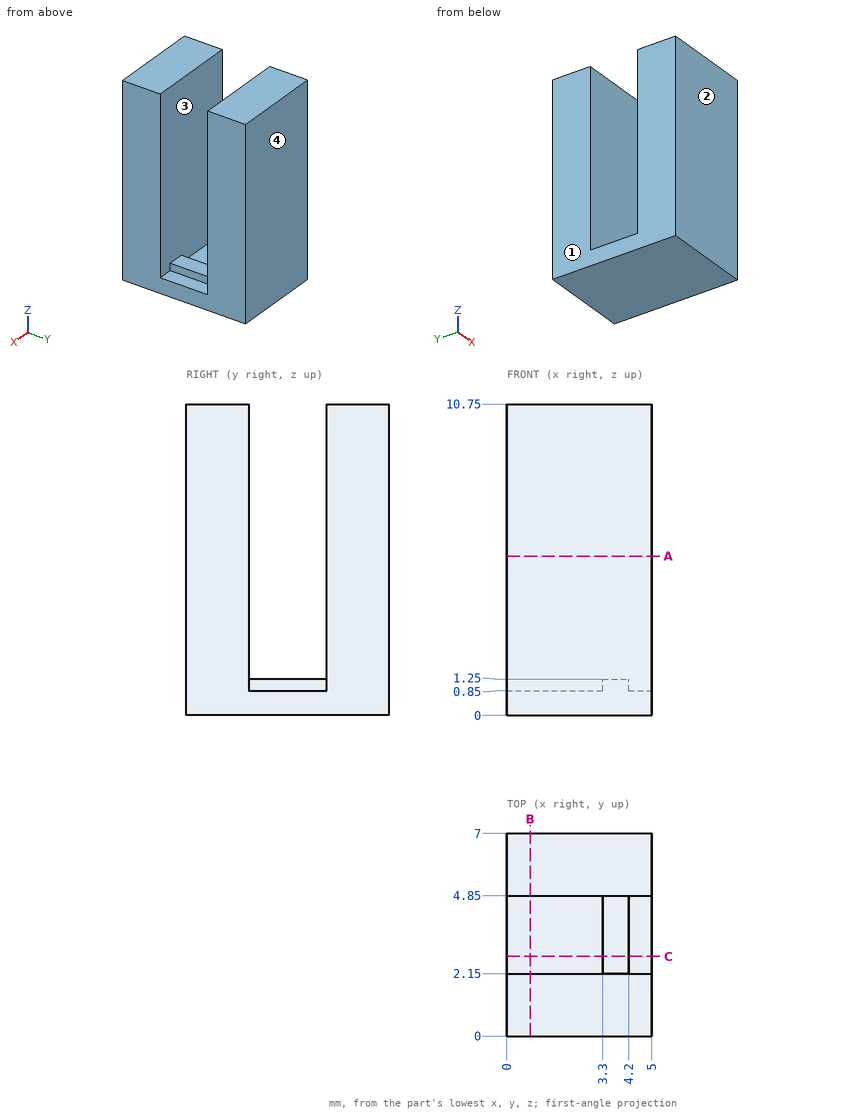
Can you work these out from the drawing? Everything is in mm from the part's minimum corner. Coordinates: 2 decimals unless noted, no trailing zeros. Order: outer loops, then holes, each group sorted by start corner. A loop starts at its lowest first (then second) coordinate and runs counter-clockwise, first axis right, second up. Notation, with made-up numbers: (-4.75, 52.25) -> (27.25, 52.25) arc R9 cw to (27.25, 58.25) -> close; hole circle Ø8 at (88, -30.5). An arc over 180 degrees is marked (long way). Use one line per item in the form item = value.
Q1. Will these pins go through, and if not, where does the flat tip stop? P1, Ø2.5, axis at x = 3.5, z = 6.5, coming from the -Y side; P2, Ø1.3, axis at x = 1.5, y = 3.5, coming from the +Z side; P3, Ø0.9, axis at x = 4.5, y = 3, coming from the +Z side.
From the geometry:
P1 = 0
P2 = 0.85
P3 = 1.25
Q2. We'd pull the mould along Y, two halves only. Please class the marked faces 1, 2, 3 and 4: released by +Y, released by -Y, zero draft, split by the parting line, or undercut.
From the geometry:
face_1 = zero draft
face_2 = released by -Y
face_3 = undercut
face_4 = released by +Y
Q3. Imagine slicing it at B-B, the plane x = 0.8. List the corners of the cut face in (y, z) for me, then the cut area to 3 significant figures.
From the geometry:
outline = (0, 0) -> (7, 0) -> (7, 10.75) -> (4.85, 10.75) -> (4.85, 0.85) -> (2.15, 0.85) -> (2.15, 10.75) -> (0, 10.75) -> close
area = 48.5 mm²
Q4. Imagine slicing it at A-A, the plane z = 5.5. List the corners of the cut face in (x, y) for me, then the cut area to 3 significant figures.
From the geometry:
outline = (0, 0) -> (5, 0) -> (5, 2.15) -> (0, 2.15) -> close; (0, 4.85) -> (5, 4.85) -> (5, 7) -> (0, 7) -> close
area = 21.5 mm²
Q5. I need wall thicknesses on L1, parallel to Y at x = 1.8, z = 9.5; L2, parallel to Z at x = 0.45, y = 4.5; L3, parallel to Z at x = 3.5, y = 3.25. Which ranges of each line are inside material? Lowest first, please.
From the geometry:
L1 = 0 to 2.15, 4.85 to 7
L2 = 0 to 0.85
L3 = 0 to 1.25
Q6. Imagine slicing it at C-C, the plane y = 2.75. List the corners of the cut face in (x, z) for me, then the cut area to 3 significant figures.
From the geometry:
outline = (0, 0) -> (5, 0) -> (5, 0.85) -> (4.2, 0.85) -> (4.2, 1.25) -> (3.3, 1.25) -> (3.3, 0.85) -> (0, 0.85) -> close
area = 4.61 mm²
